Print and shaded views of the part. All mm, measured from the part's lowest x, y and z. A direction names the side the tool comes from. Give positions to 0.01 mm unless a question says otherwise; leave off trailing zeros. Loops run counter-clockwise (first coordinate to the right, second up) from the corner with the lowest first, then second, coordinate; pieces in that order, holes last.
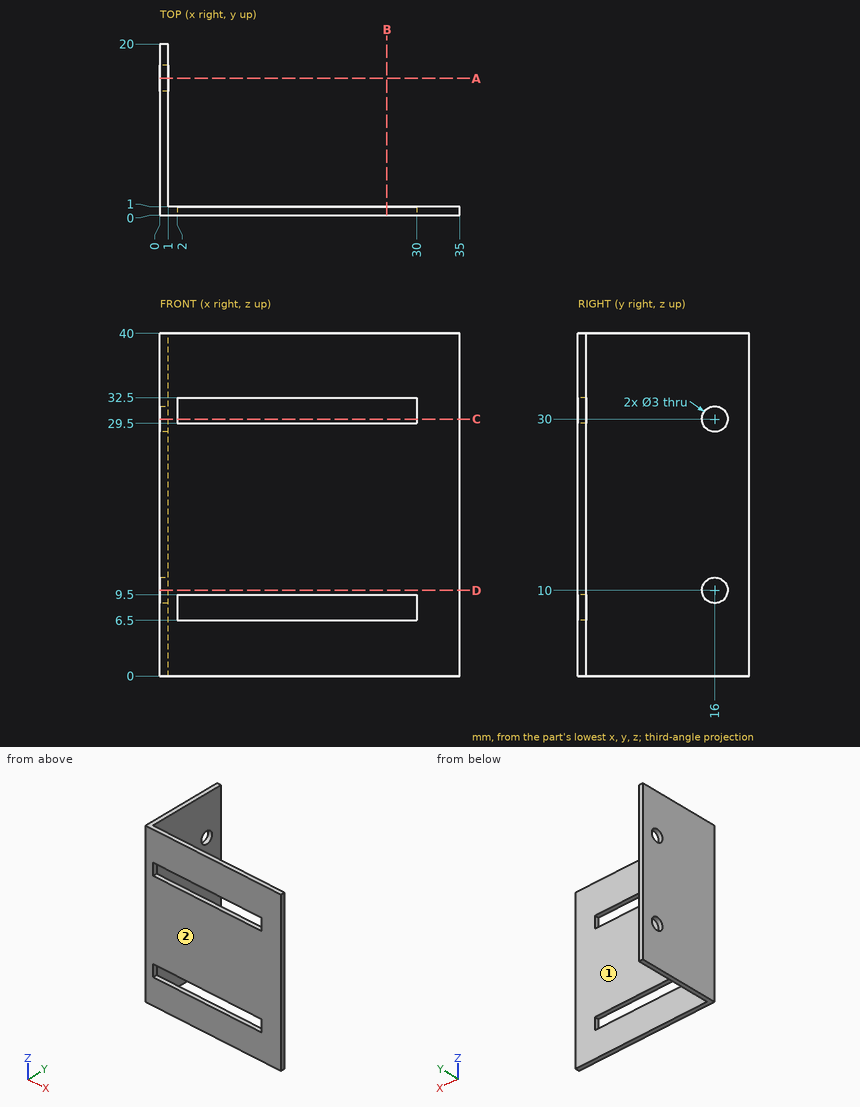
1. Tool access for the marked faces 1 and 2: list every direction of +Z, -Z, +X, -X, +Y, -Y with a clear straight run to the whole face (end or side of a thin tool).
Responses:
face 1: +Z, -Z, +X, +Y
face 2: +Z, -Z, +X, -X, -Y
2. Saw through at D-D, the plane z = 10. List the corners of the cut face in (x, y), and give its area (3 significant figures).
Responses:
outline: (0, 0) - (35, 0) - (35, 1) - (1, 1) - (1, 14.5) - (0, 14.5) - close; (0, 17.5) - (1, 17.5) - (1, 20) - (0, 20) - close
area: 51.0 mm2
3. Saw through at A-A, the plane y = 16. List the corners of the cut face in (x, z).
Responses:
outline: (0, 0) - (1, 0) - (1, 8.5) - (0, 8.5) - close; (0, 11.5) - (1, 11.5) - (1, 28.5) - (0, 28.5) - close; (0, 31.5) - (1, 31.5) - (1, 40) - (0, 40) - close
4. Probe line 1 along Y through (x, z) = (0.7, 30); line 2 along X through (y, z) = (16, 12). List the from-to ranges inside material, lowest first.
Responses:
line 1: y = 0 to 14.5, 17.5 to 20
line 2: x = 0 to 1
5. Saw through at C-C, the plane z = 30. List the corners of the cut face in (x, y).
Responses:
outline: (0, 0) - (2, 0) - (2, 1) - (1, 1) - (1, 14.5) - (0, 14.5) - close; (0, 17.5) - (1, 17.5) - (1, 20) - (0, 20) - close; (30, 0) - (35, 0) - (35, 1) - (30, 1) - close
6. Drop flat-ended pins along their axis: pin 1 (5.5 mm diameter, centred on y = 10.5, z = 15.5, fed in from +X); pin 2 (2.5 mm diameter, centred on y = 16, z = 30, fed in from +X); pin 3 (3 mm diameter, centred on y = 13.5, z = 22, fed in from -X); pin 4 (12 mm diameter, centred on x = 15, z = 10, fed in from +Y). Give the stop position or say it passes through.
Responses:
pin 1: stops at x = 1
pin 2: passes through
pin 3: stops at x = 0
pin 4: stops at y = 1
7. Saw through at B-B, the plane x = 26.5. List the corners of the cut face in (y, z).
Responses:
outline: (0, 0) - (1, 0) - (1, 6.5) - (0, 6.5) - close; (0, 9.5) - (1, 9.5) - (1, 29.5) - (0, 29.5) - close; (0, 32.5) - (1, 32.5) - (1, 40) - (0, 40) - close
